Verification items for the finished model (mm, model axes). Give positions to 0.01 mm unless a question says otherwise; leave off trailing zeros. Write each loop counter-clockwise with the first axis right and the second up, starting at its lowest first coordinate (ties: lowest second). Pieces come first, ordered by that corner, then holes.
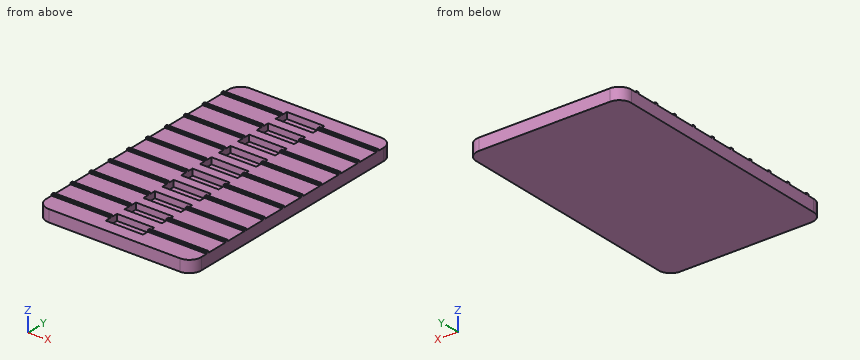
from build123d import *

# Parameters (mm, degrees)
F0_W     = 49.53
F0_H     = 81.28
F1_DEPTH = 3.81
F2_W     = 11.938
F2_H     = 4.572
F3_DEPTH = 2.032
F4_W     = 18.796
F4_H     = 0.762
F5_DEPTH = 0.508
F6_R     = 3.81


with BuildPart() as f1:
    # F0 (on Top) → F1 (new body)
    with BuildSketch(Plane.XY):
        with Locations((24.765, 40.64)):
            Rectangle(F0_W, F0_H)
    extrude(amount=F1_DEPTH)

    # F2 (on face) → F3 (cut)
    with BuildSketch(Plane.XY.offset(3.81)):
        with Locations((24.765, 6.35)):
            Rectangle(F2_W, F2_H)
        with Locations((24.765, 13.97)):
            Rectangle(F2_W, F2_H)
        with Locations((24.765, 21.59)):
            Rectangle(F2_W, F2_H)
        with Locations((24.765, 29.21)):
            Rectangle(F2_W, F2_H)
        with Locations((24.765, 36.83)):
            Rectangle(F2_W, F2_H)
        with Locations((24.765, 44.45)):
            Rectangle(F2_W, F2_H)
        with Locations((24.765, 52.07)):
            Rectangle(F2_W, F2_H)
        with Locations((24.765, 59.69)):
            Rectangle(F2_W, F2_H)
        with Locations((24.765, 67.31)):
            Rectangle(F2_W, F2_H)
        with Locations((24.765, 74.93)):
            Rectangle(F2_W, F2_H)
    extrude(amount=-F3_DEPTH, mode=Mode.SUBTRACT)

    # F4 (on face) → F5 (join)
    with BuildSketch(Plane.XY.offset(3.81)):
        with Locations((40.132, 6.35)):
            Rectangle(F4_W, F4_H)
        with Locations((9.398, 6.35)):
            Rectangle(F4_W, F4_H)
        with Locations((9.398, 13.97)):
            Rectangle(F4_W, F4_H)
        with Locations((40.132, 13.97)):
            Rectangle(F4_W, F4_H)
        with Locations((9.398, 21.59)):
            Rectangle(F4_W, F4_H)
        with Locations((40.132, 21.59)):
            Rectangle(F4_W, F4_H)
        with Locations((9.398, 29.21)):
            Rectangle(F4_W, F4_H)
        with Locations((40.132, 29.21)):
            Rectangle(F4_W, F4_H)
        with Locations((9.398, 36.83)):
            Rectangle(F4_W, F4_H)
        with Locations((40.132, 36.83)):
            Rectangle(F4_W, F4_H)
        with Locations((9.398, 44.45)):
            Rectangle(F4_W, F4_H)
        with Locations((40.132, 44.45)):
            Rectangle(F4_W, F4_H)
        with Locations((9.398, 52.07)):
            Rectangle(F4_W, F4_H)
        with Locations((40.132, 52.07)):
            Rectangle(F4_W, F4_H)
        with Locations((9.398, 59.69)):
            Rectangle(F4_W, F4_H)
        with Locations((40.132, 59.69)):
            Rectangle(F4_W, F4_H)
        with Locations((9.398, 67.31)):
            Rectangle(F4_W, F4_H)
        with Locations((40.132, 67.31)):
            Rectangle(F4_W, F4_H)
        with Locations((9.398, 74.93)):
            Rectangle(F4_W, F4_H)
        with Locations((40.132, 74.93)):
            Rectangle(F4_W, F4_H)
    extrude(amount=F5_DEPTH)

    # F6
    f6_edges = [f1.edges().sort_by_distance(p)[0] for p in [
        (49.53, 0, 1.905),
        (0, 0, 1.905),
        (0, 81.28, 1.905),
        (49.53, 81.28, 1.905),
    ]]
    fillet(f6_edges, radius=F6_R)


solid = f1.part
Item 1: Depth check by flat-ended pin: pin 1 (6 mm diameter, centred on x = 12.5, y = 46.5, fed in from +Z); pin 2 (6 mm diameter, centred on x = 22, y = 39.5, fed in from +Z). Enter the tip coordinate at first touch or a pass-through.
Answer key:
pin 1: stops at z = 4.32
pin 2: stops at z = 3.81
Item 2: Scan lines: line 1 along X through (y, z) = (66, 2.2); line 2 along Z through (x, y) = (28.5, 63.5); line 3 along Z through (x, y) = (23, 35). Record each from-to range of solid material in increasing order.
Answer key:
line 1: x = 0 to 18.8, 30.73 to 49.53
line 2: z = 0 to 3.81
line 3: z = 0 to 1.78
Item 3: Sectioned sample at B-B on z = 2.9. State how many separate pieces and enclosed holes the cut face has, then the cut area to 3 significant figures.
Answer key:
separate pieces: 1
enclosed holes: 10
area: 3,470 mm2
Item 4: Sectioned sample at A-A on y = 28. Record the cut outline in (x, z).
Answer key:
outline: (0, 0) - (49.53, 0) - (49.53, 3.81) - (30.73, 3.81) - (30.73, 1.78) - (18.8, 1.78) - (18.8, 3.81) - (0, 3.81) - close
